Read the model definition and answer for the solid it produces. Units are mm, in the model's axes. Give positions to 0.01 mm unless a question says otherwise; leave off trailing zeros. Loops run counter-clockwise (first coordinate to the right, second up) from the corner with the lowest first, then second, coordinate; pieces in that order, holes last. Notation, with made-up numbers: (-3, 15) - (18, 15) arc R11 cw to (18, 27) - close; hole circle Ø3 at (0, 18). An arc over 180 degrees is marked (long way). Use a Markdown table: item, result. Add a question column.
Item 1: Each of these flat-tipped pins is pushed along its axis until it touches: P1, Ø2.5, axis at x = 0, z = 35, coming from the +Y side; P2, Ø3, axis at x = 2, y = -2, coming from the -Z side. Where does it stop, or does it pass through?
Item 2: A cutting plane is placed at D-D (y = 0.45). Determine the outline of the cut face in (x, z), plus the area to 3 significant figures.
Item 3: A cutting plane is placed at A-A (x = 0). Determine the outline of the cut face in (y, z).
Item 4: For a pull along Z with two mould halves and no side action, classify faces 1 (the face through (-0.325, 0.042, 36.464)), 2 (the face through (0, -3, 20)), 3 (the face through (0, 0, 40)) as +Z half, -Z half, draft (parallel to the pull), parting line (faces both ways), or undercut.
Item 5: A cutting plane is placed at B-B (z = 15). Determine the outline of the cut face in (x, y), plus the area to 3 significant figures.
Item 6: Consider probe 1 along Y at (x, z) = (-0.3, 5); probe 2 along Z at (x, y) = (2.1, 1.1); probe 3 along Z at (x, y) = (-0.3, -2.15). Determine where each line is inside the solid, lowest interval first. Write a range as [from, to].
Item 7: A cutting plane is placed at C-C (y = 2.3). Determine the outline of the cut face in (x, z), plus the area to 3 significant figures.
from build123d import *

# Parameters (mm, degrees)
SKETCH_1_W          = 6
SKETCH_1_H          = 6
EXTRUDE_1_DEPTH     = 40
SKETCH_2_R          = 1.5
CUT_EXTRUDE_1_DEPTH = 7
SKETCH_3_R          = 1.5
CUT_EXTRUDE_2_DEPTH = 7


with BuildPart() as part:
    # 草图1 → 凸台-拉伸1 (new body)
    with BuildSketch(Plane.XY):
        Rectangle(SKETCH_1_W, SKETCH_1_H)
    extrude(amount=EXTRUDE_1_DEPTH)

    # 草图2 → 切除-拉伸1 (cut, through all)
    with BuildSketch(Plane.ZY.offset(3)):
        with Locations((5, 0)):
            Circle(SKETCH_2_R)
        with Locations((25, 0)):
            Circle(SKETCH_2_R)
    extrude(amount=-CUT_EXTRUDE_1_DEPTH, mode=Mode.SUBTRACT)

    # 草图3 → 切除-拉伸2 (cut, through all)
    with BuildSketch(Plane(origin=(0, 3, 0), x_dir=(1, 0, 0), z_dir=(0, 1, 0))):
        with Locations((0, -15)):
            Circle(SKETCH_3_R)
        with Locations((0, -35)):
            Circle(SKETCH_3_R)
    extrude(amount=-CUT_EXTRUDE_2_DEPTH, mode=Mode.SUBTRACT)


solid = part.part
Geometry says:
| question | item | result |
|---|---|---|
| 1 | P1 | through |
| 1 | P2 | z = 0 |
| 2 | outline | (-3, 0) - (3, 0) - (3, 3.57) - (-3, 3.57) - close; (-3, 6.43) - (3, 6.43) - (3, 23.57) - (-3, 23.57) - close; (-3, 26.43) - (3, 26.43) - (3, 40) - (-3, 40) - close; hole circle Ø3 at (0, 15); hole circle Ø3 at (0, 35) |
| 2 | area | 192 mm² |
| 3 | outline | (-3, 0) - (3, 0) - (3, 13.5) - (-3, 13.5) - close; (-3, 16.5) - (3, 16.5) - (3, 33.5) - (-3, 33.5) - close; (-3, 36.5) - (3, 36.5) - (3, 40) - (-3, 40) - close; hole circle Ø3 at (0, 5); hole circle Ø3 at (0, 25) |
| 4 | face 1 | undercut |
| 4 | face 2 | draft |
| 4 | face 3 | +Z half |
| 5 | outline | (-3, -3) - (-1.5, -3) - (-1.5, 3) - (-3, 3) - close; (1.5, -3) - (3, -3) - (3, 3) - (1.5, 3) - close |
| 5 | area | 18.0 mm² |
| 6 | probe 1 | [-3, -1.5], [1.5, 3] |
| 6 | probe 2 | [0, 3.98], [6.02, 23.98], [26.02, 40] |
| 6 | probe 3 | [0, 13.53], [16.47, 33.53], [36.47, 40] |
| 7 | outline | (-3, 0) - (3, 0) - (3, 40) - (-3, 40) - close; hole circle Ø3 at (0, 15); hole circle Ø3 at (0, 35) |
| 7 | area | 226 mm² |
